Input: part model. Units: mm. Frame: model coordinates. Give positions to 0.01 mm unless a question says otherwise; leave off trailing zeros. Loops run counter-clockwise (first coordinate to the right, second up) from the corner with the lowest first, then second, coordinate; pieces in that order, holes last. Notation, with made-up numbers: M -19,57.5 L -2,57.5 A25 cw -2,72.5 Z; hole C 43.25,25 d5. An arc over 180 degrees is marked long. One line per item, written item: value. Start each with the question number.
(1) Section A-A on z = 3. Output: boundary loops of the cut face in (x, y), plus the area to 3 significant figures.
(2) Ray query, line 1 along X through (y, z) = (-0.5, 6.5); line 2 along X through (y, z) = (5.5, 5.5). Return the intervals inside material, ascending. Write a range as from..to.
(3) Section C-C on y = 4.75. Output: boundary loops of the cut face in (x, z), plus the area to 3 significant figures.
(4) Pin query (flat end, axial travel): P1, Ø5, axis at y = -4.5, z = 9, coming from the -X side. Return the tip coordinate at first contact, or that it passes through.
(5) Section B-B on y = -4.5. Output: boundary loops of the cut face in (x, z), plus the area to 3 significant figures.
```python
from build123d import *

# Parameters (mm, degrees)
F1_DEPTH = 11.4


with BuildPart() as f1:
    # F0 (on Top) → F1 (new body)
    with BuildSketch(Plane.XY):
        with BuildLine():
            ThreePointArc((0, 8.5), (6.010408, 6.010408), (8.5, 0))
            ThreePointArc((8.5, 0), (6.010408, -6.010408), (0, -8.5))
            Line((0, -8.5), (83, -8.5))
            ThreePointArc((83, -8.5), (74.5, 0), (83, 8.5))
            Line((83, 8.5), (0, 8.5))
        make_face()
        with BuildLine():
            ThreePointArc((0, -8.5), (6.010408, -6.010408), (8.5, 0))
            ThreePointArc((8.5, 0), (6.010408, 6.010408), (0, 8.5))
            ThreePointArc((0, 8.5), (-8.5, 0), (0, -8.5))
        make_face()
        with BuildLine():
            ThreePointArc((91.5, 0), (89.010408, 6.010408), (83, 8.5))
            ThreePointArc((83, 8.5), (74.5, 0), (83, -8.5))
            ThreePointArc((83, -8.5), (89.010408, -6.010408), (91.5, 0))
        make_face()
    extrude(amount=F1_DEPTH)


solid = f1.part
```
Output values:
1. outline: M 0,-8.5 L 83,-8.5 A8.5 ccw 91.5,0 A8.5 ccw 83,8.5 L 0,8.5 A8.5 ccw Z
1. area: 1,640 mm²
2. line 1: x = -8.49..91.49
2. line 2: x = -6.48..89.48
3. outline: M -7.05,0 L 90.05,0 L 90.05,11.4 L -7.05,11.4 Z
3. area: 1,110 mm²
4. P1: stops at x = -8.26
5. outline: M -7.21,0 L 90.21,0 L 90.21,11.4 L -7.21,11.4 Z
5. area: 1,110 mm²
